Geometry: see drawing. Coordinates: mm, zero at the bounding-box minimum. A direction names the side the tool comes from. Give positions to 0.01 mm unless a question says otherwise; leave off trailing zeros. Loops run counter-clockwise (first coordinate to the right, second up) from the corner with the lowest first, then second, coordinate; pieces in that order, holes last. Notation, with made-up numbers: M -19,14 L -5,14 A10 cw -5,32 Z; hole C -28.5,47.5 d3. An arc over 180 degrees is marked long. Put each result on its own line as item: value.
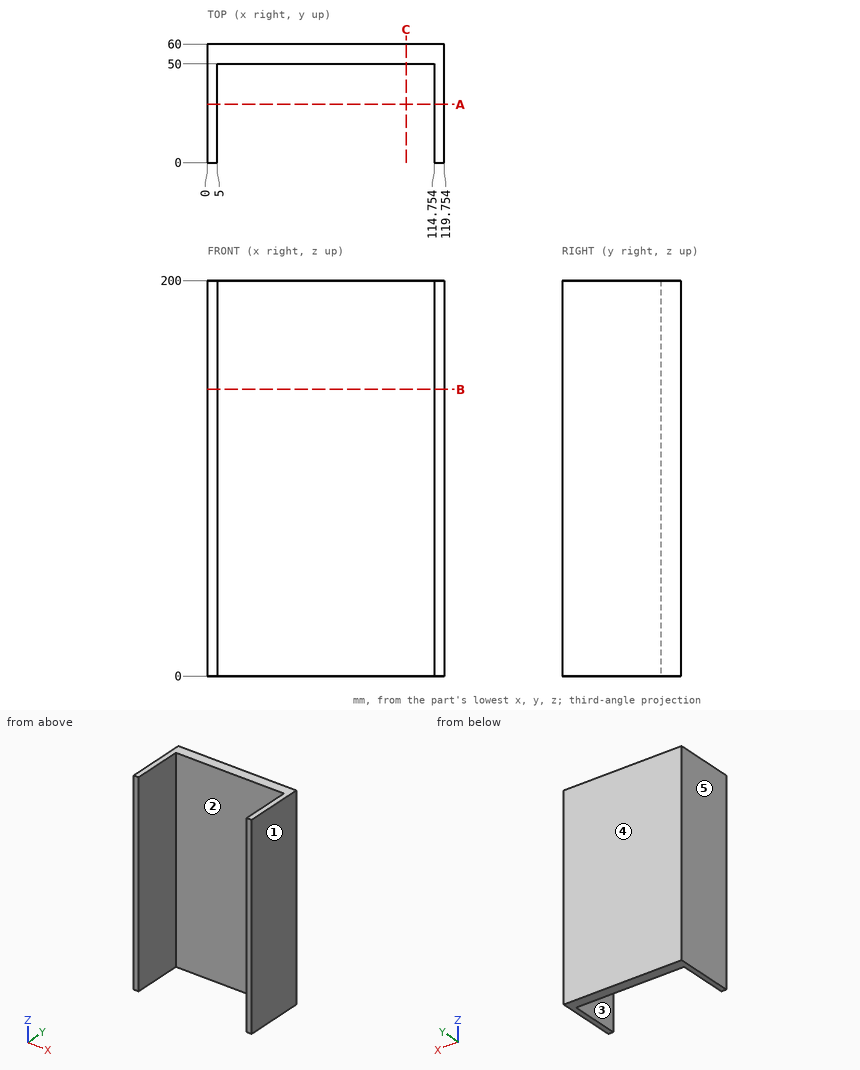
1. Material intervals for line 1 (X direction, y = 25, z = 59); line 2 (Y direction, x = 39.5, z = 120), sorted ascending. Write a range as from..to.
Found:
line 1: 0..5, 114.75..119.75
line 2: 50..60
2. Section query B-B (z = 145). Output: boundary loops of the cut face in (x, y).
Found:
outline: M 0,0 L 5,0 L 5,50 L 114.75,50 L 114.75,0 L 119.75,0 L 119.75,60 L 0,60 Z
3. Contact query for flat-ended pins moving along their axis: P1, Ø1, axis at x = 97.5, z = 160, coming from the -Y side; P2, Ø12, axis at x = 103.5, y = 32.5, coming from the -Z side. Output: stop coordinate, or through.
Found:
P1: y = 50
P2: through
4. Section query C-C (x = 100.5). Output: boundary loops of the cut face in (y, z).
Found:
outline: M 50,0 L 60,0 L 60,200 L 50,200 Z
5. Draft query along X for the marked faces 3, 4 and 5. Return one class per face: pulls with the +X half, pulls with the -X half, needs draft (parallel to the pull), parting line crosses it, or undercut.
Found:
face 3: undercut
face 4: needs draft
face 5: pulls with the -X half
6. Section query A-A (y = 29.5). Output: boundary loops of the cut face in (x, z).
Found:
outline: M 0,0 L 5,0 L 5,200 L 0,200 Z; M 114.75,0 L 119.75,0 L 119.75,200 L 114.75,200 Z
7. Access query for the marked faces 1 and 2. Directions: +Z, -Z, +X, -X, +Y, -Y. A direction counts if a zero-diameter tool reaches every point of the face in a straight line with its end or side. Return the directions, or none.
Found:
face 1: +Z, -Z, +X, +Y, -Y
face 2: +Z, -Z, -Y
